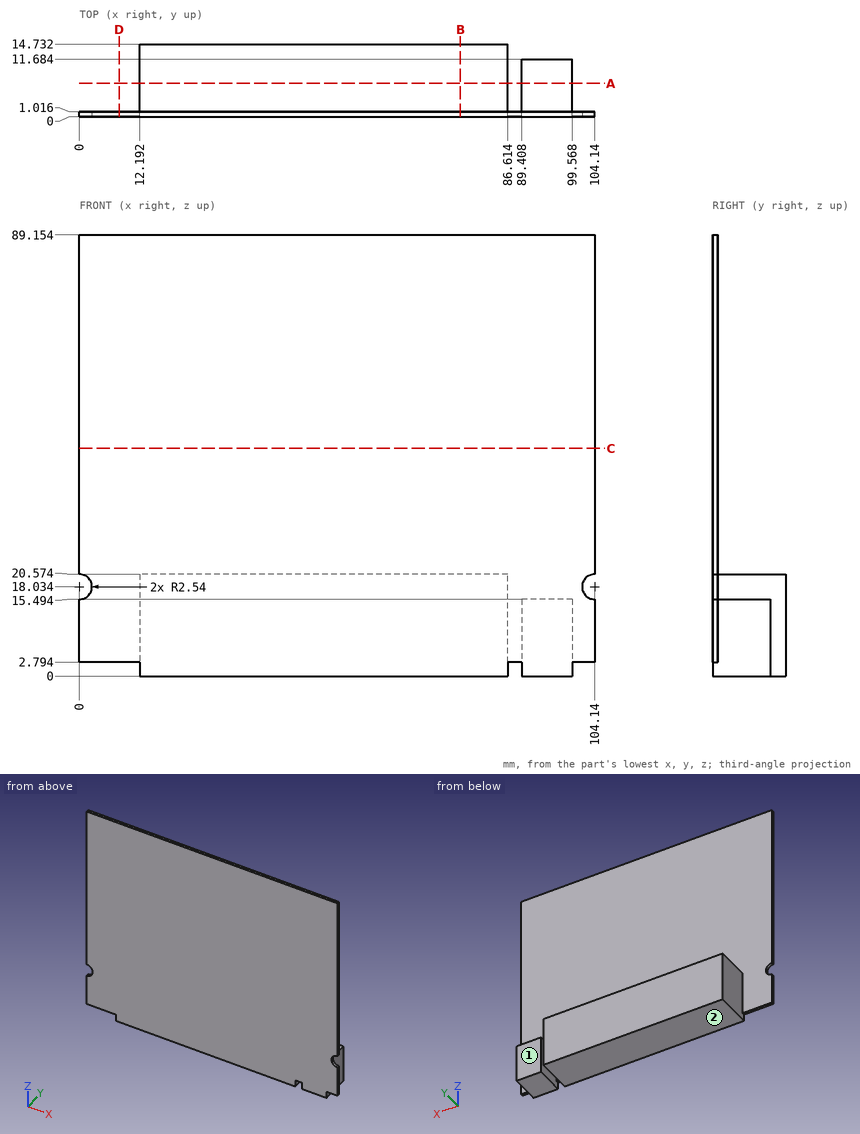
Geometry check sheet. Reference: drawing and pictorial views, mm from the part's lowest x, y, z. A direction names the side the tool comes from. Round coordinates to 2 decimals unless told otherwise and drop trailing zeros. Write each loop counter-clockwise with the first axis right and the second up, starting at its lowest first coordinate (ties: lowest second). Pieces come first, ordered by that corner, then holes.
(1) Access from +Z, -Z, +X, -X, +Y, -Y to the whole of each face (thin tool, end or side, straight path). Record for the marked faces 1 and 2.
Returned:
face 1: +Z, -Z, +X, +Y
face 2: -Z, +X, -X, +Y, -Y
(2) Section check D-D (x = 8). Enter the section's corners in (y, z), plus the area to 3 significant figures.
Returned:
outline: (0, 2.79) - (1.02, 2.79) - (1.02, 89.15) - (0, 89.15) - close
area: 87.7 mm2
(3) Material ranges on line 1 (X direction, y = 8, z = 12.5); line 2 (Y direction, x = 44, z = 69); line 3 (Z direction, x = 64.5, y = 11.5), recorded low to high.
Returned:
line 1: x = 12.19 to 86.61, 89.41 to 99.57
line 2: y = 0 to 1.02
line 3: z = 0 to 20.57
(4) Section check C-C (z = 46). Enter the section's corners in (x, y).
Returned:
outline: (0, 0) - (104.14, 0) - (104.14, 1.02) - (0, 1.02) - close
(5) Section check B-B (x = 77). Enter the section's corners in (y, z), plus the area to 3 significant figures.
Returned:
outline: (0, 0) - (14.73, 0) - (14.73, 20.57) - (1.02, 20.57) - (1.02, 89.15) - (0, 89.15) - close
area: 373 mm2
(6) Section check A-A (y = 6.75). Enter the section's corners in (x, z), plus the area to 3 significant figures.
Returned:
outline: (12.19, 0) - (86.61, 0) - (86.61, 20.57) - (12.19, 20.57) - close; (89.41, 0) - (99.57, 0) - (99.57, 15.49) - (89.41, 15.49) - close
area: 1,690 mm2
(7) Depth check by flat-ended pin: pin 1 Ø0.5 at (x, y) = (102.5, 0.5) entering from -Z; pin 2 Ø4.5 at (y, z) = (4, 6) entering from +X; pin 3 Ø4.5 at (y, z) = (8, 7) entering from -X. Enter the tip coordinate at first touch or a pass-through.
Returned:
pin 1: stops at z = 2.79
pin 2: stops at x = 99.57
pin 3: stops at x = 12.19
